Autodesk Inventor part; units mm, degrees
ref_plane "YZ Plane" through (0, 0, 0) normal (1, 0, 0) x (0, 1, 0)
ref_plane "XZ Plane" through (0, 0, 0) normal (0, 1, 0) x (-1, 0, 0)
ref_plane "XY Plane" through (0, 0, 0) normal (0, 0, 1) x (1, 0, 0)
sketch "Sketch1" plane through (0, 0, 0) normal (0, 0, 1) x (1, 0, 0)
  line L0 (0, 0) -> (71.1, 0)
  line L1 (71.1, 0) -> (71.1, 71.1)
  line L2 (71.1, 71.1) -> (0, 71.1)
  line L3 (0, 71.1) -> (0, 0)
  circle A0 centre (35.55, 35.55) radius 24.15
  dimension "d0" = 71.1
  dimension "d1" = 71.1
  dimension "d2" = 48.3
extrude "Extrusion1" add sketch "Sketch1" along normal blind 12.7
sketch "Sketch2" plane through (0, 0, 12.7) normal (0, 0, 1) x (1, 0, 0)
  line L0 (71.1, 71.1) -> (0, 71.1)
  line L1 (0, 71.1) -> (0, 0)
  line L2 (0, 0) -> (71.1, 0)
  line L3 (71.1, 0) -> (71.1, 71.1)
  circle A0 centre (35.55, 35.55) radius 24.15
  circle A1 centre (35.55, 35.55) radius 24.15
  circle A2 centre (35.55, 35.55) radius 32.4
  dimension "d5" = 64.8
extrude "Extrusion2" add sketch "Sketch2" along normal blind 7.9 contours A2
sketch "Sketch3" plane through (0, 71.1, 0) normal (0, 1, 0) x (1, 0, 0)
  line L0 (71.1, 0) -> (0, 0)
  line L1 (0, 0) -> (0, -12.7)
  line L2 (71.1, -12.7) -> (0, -12.7)
  line L3 (71.1, 0) -> (71.1, -12.7)
  line L4 (71.1, 0) -> (71.1, -12.7)
  line L5 (71.1, -12.7) -> (35.55, -12.7)
  line L6 (0, -12.7) -> (71.1, -12.7)
  line L7 (35.55, -12.7) -> (20.55, -12.7)
  line L8 (20.55, -12.7) -> (23.7, -12.7)
  arc A0 (23.7, -9.55) -> (20.55, -12.7) centre (23.7, -12.7) ccw
  line L9 (35.55, -12.7) -> (47.4, -12.7)
  arc A1 (50.55, -12.7) -> (47.4, -9.55) centre (47.4, -12.7) ccw
  line L10 (47.4, -9.55) -> (23.7, -9.55)
  dimension "d8" = 35.55
  dimension "d9" = 15
  dimension "d10" = 3.15
  dimension "d11" = 11.85
  dimension "d12" = 6.3
revolve "Revolution1" cut sketch "Sketch3" angle 360 about axis through (71.1, 71.1, 12.7) along (-1, 0, 0) contours L2 A0 L10 A1
sketch "Sketch4" plane through (0, 0, 12.7) normal (0, 0, 1) x (1, 0, 0)
  arc A0 (20.55, 71.1) -> (23.7, 67.95) centre (23.7, 71.1) ccw
  line L0 (20.55, 71.1) -> (0, 71.1)
  line L1 (0, 71.1) -> (0, 0)
  line L2 (0, 0) -> (71.1, 0)
  line L3 (71.1, 0) -> (71.1, 71.1)
  line L4 (71.1, 71.1) -> (50.55, 71.1)
  arc A1 (47.4, 67.95) -> (50.55, 71.1) centre (47.4, 71.1) ccw
  line L5 (47.4, 67.95) -> (35.55, 67.95)
  circle A2 centre (35.55, 35.55) radius 32.4
  line L6 (35.55, 67.95) -> (23.7, 67.95)
  line L7 (35.55, 35.55) -> (65.55, 35.55)
  line L8 (65.55, 35.55) -> (65.55, 65.55)
  line L9 (65.55, 65.55) -> (5.55, 65.55)
  line L10 (5.55, 65.55) -> (5.55, 5.55)
  line L11 (5.55, 5.55) -> (65.55, 5.55)
  circle A3 centre (65.55, 65.55) radius 3
  circle A4 centre (5.55, 65.55) radius 3
  circle A5 centre (5.55, 5.55) radius 3
  circle A6 centre (65.55, 5.55) radius 3
  dimension "d14" = 30
  dimension "d15" = 30
  dimension "d16" = 60
  dimension "d17" = 60
  dimension "d18" = 60
  dimension "d19" = 6
  dimension "d20" = 6
  dimension "d21" = 6
  dimension "d22" = 6
extrude "Extrusion3" cut sketch "Sketch4" against normal blind 12.7 contours A6 | A3 L8 L9 | L9 L8 A3 | A4 L10 L9 | L9 L10 A4 | A5 L11 L10 | L10 L11 A5
sketch "Sketch5" plane through (71.1, 0, 0) normal (1, 0, 0) x (0, 0, -1)
  line L0 (0, 0) -> (0, 71.1)
  line L1 (0, 71.1) -> (-12.7, 71.1)
  line L2 (-12.7, 0) -> (-12.7, 71.1)
  line L3 (0, 0) -> (-12.7, 0)
  line L4 (-12.7, 71.1) -> (-12.7, 0)
  line L5 (-12.7, 35.55) -> (-6.35, 35.55)
  circle A0 centre (-6.35, 35.55) radius 1
  line L6 (-6.35, 35.55) -> (-9.525, 35.55)
  line L7 (-9.525, 35.55) -> (-9.525, 65.55)
  line L8 (-9.525, 65.55) -> (-9.525, 61.97)
  line L9 (-9.525, 65.55) -> (-3.175, 65.55)
  line L10 (-3.175, 65.55) -> (-3.175, 5.55)
  line L11 (-3.175, 5.55) -> (-3.175, 9.13)
  line L12 (-3.175, 9.13) -> (-9.525, 9.13)
  circle A1 centre (-9.525, 9.13) radius 0.65
  circle A2 centre (-3.175, 9.13) radius 0.65
  circle A3 centre (-9.525, 61.97) radius 0.65
  circle A4 centre (-3.175, 61.97) radius 0.65
  line L13 (-9.525, 61.97) -> (-3.175, 61.97)
  dimension "d25" = 6.35
  dimension "d26" = 2
  dimension "d37" = 3.175
  dimension "d38" = 30
  dimension "d39" = 3.58
  dimension "d40" = 6.35
  dimension "d41" = 60
  dimension "d42" = 3.58
  dimension "d43" = 6.35
  dimension "d44" = 1.3
  dimension "d45" = 1.3
  dimension "d46" = 1.3
  dimension "d47" = 1.3
  dimension "d48" = 6.35
extrude "Extrusion4" cut sketch "Sketch5" against normal blind 4.75 contours A1 | A2 L10 | L10 L12 A2 | A3 L7 | L7 L13 A3 | A0 | L7 A3 L13 | L13 L10 A4 | A4 L10 L13 | A4 L10 | L10 A2 L12
sketch "Sketch6" plane through (0, 0, 0) normal (0, -1, 0) x (1, 0, 0)
  line L0 (0, 0) -> (71.1, 0)
  line L1 (71.1, 0) -> (71.1, 12.7)
  line L2 (0, 12.7) -> (71.1, 12.7)
  line L3 (0, 0) -> (0, 12.7)
  circle A0 centre (35.55, 6.35) radius 2
  dimension "d29" = 4
extrude "Extrusion5" cut sketch "Sketch6" against normal blind 6.1 contours A0
thread "Thread1"
chamfer "Chamfer1" distance 2.55 angle 45 4 edges at (71.1, 71.1, 6.35) (71.1, 0, 6.35) (0, 71.1, 6.35) (0, 0, 6.35)
sketch "Sketch7" plane through (0, 2.55, 0) normal (-1, 0, 0) x (0, 0, 1)
  circle A0 centre (9.525, 6.58) radius 0.65
  circle A1 centre (3.175, 6.58) radius 0.65
  circle A2 centre (3.175, 59.42) radius 0.65
  circle A3 centre (6.35, 33) radius 1
  circle A4 centre (9.525, 59.42) radius 0.65
  line L0 (0, 0) -> (12.7, 0)
  line L1 (0, 0) -> (0, 66)
  line L2 (12.7, 66) -> (0, 66)
  line L3 (12.7, 0) -> (12.7, 66)
  circle A5 centre (3.175, 59.42) radius 0.65
  circle A6 centre (9.525, 59.42) radius 0.65
  circle A7 centre (6.35, 33) radius 1
  circle A8 centre (3.175, 6.58) radius 0.65
  circle A9 centre (3.175, 6.58) radius 0.65
  circle A10 centre (9.525, 6.58) radius 0.65
  point P0 (0, -2.55)
  dimension "d49" = 1.3
  dimension "d50" = 1.3
  dimension "d51" = 2
  dimension "d52" = 1.3
  dimension "d53" = 1.3
extrude "Extrusion6" cut sketch "Sketch7" against normal blind 4.75 contours A0 | A1 | A2 | A3 | A4
properties part number "0x001" material "Iron, Cast"
Work out the finished part from the listing and answer in its coordinate system (mm). A direction names the side the tool comes from. Coordinates: 2 decimals unless noted, no trailing zeros. Write each loop counter-clockwise with the first axis right and the second up, starting at its lowest first coordinate (ties: lowest second). Pieces come first, ordered by that corner, then holes.
Q1. A cutting plane is placed at D-D, the plane y = 65.55. Give the vertices of the cut face in (x, z), then the cut area to 3 significant figures.
Q2. Determine the mould class of faces 1 (the face through (66.454, 25.818, 16.595)), 2 (the face through (2.342, 34.574, 6.133)), 3 (the face through (4.9, 62.62, 6.44)), 4 (the face through (11, 36, 0)) for opening direction Y: released by +Y, released by -Y, zero draft, split by the parting line, or undercut.
Q3. A cutting plane is placed at C-C, the plane y = 39. Give the vertices of the cut face in (x, z).
Q4. Which of the six approach directions +Z, -Z, +X, -X, +Y, -Y give full straight-line access (tool end or side, diameter ignored) to faces 5 (the face through (35.384, 68.897, 10.448)), 6 (the face through (36, 6.1, 6)), 7 (the face through (25, 4, 12.7)), 8 (the face through (4.75, 36, 6))?
Q5. A cutting plane is placed at B-B, the plane x = 58.5. Give the vertices of the cut face in (y, z), then the cut area to 3 significant figures.
Q6. Find the intervals of material crossed by line 1 (X direction, y = 65.55, z = 9); line 2 (Z direction, x = 1, y = 9); line 3 (Z direction, x = 68.5, y = 63), in increasing order.
Q7. Each of these flat-tipped pins is pushed along its axis until it touches: pin 1 Ø8 at (x, z) = (21.5, 10) entering from -Y; pin 2 Ø0.6 at (y, z) = (35.5, 6) entering from -X; pin 3 Ø3 at (y, z) = (15.5, 18) entering from -X; pin 4 Ø0.8 at (y, z) = (61.97, 9.525) entering from +X. Where does it stop, or does it pass through?
Q8. A cutting plane is placed at A-A, the plane z = 6.35. Give the vertices of the cut face in (x, y).
Findings below:
1. outline: (0, 0) - (2.55, 0) - (2.55, 12.7) - (0, 12.7) - close; (8.55, 0) - (62.55, 0) - (62.55, 12.7) - (47.79, 12.7) - (47.79, 20.6) - (23.31, 20.6) - (23.31, 12.7) - (8.55, 12.7) - close; (68.55, 0) - (71.1, 0) - (71.1, 12.7) - (68.55, 12.7) - close
1. area: 944 mm2
2. face 1: split by the parting line
2. face 2: undercut
2. face 3: undercut
2. face 4: zero draft
3. outline: (0, 0) - (11.65, 0) - (11.65, 20.6) - (3.33, 20.6) - (3.33, 12.7) - (0, 12.7) - close; (59.45, 0) - (71.1, 0) - (71.1, 12.7) - (67.77, 12.7) - (67.77, 20.6) - (59.45, 20.6) - close
4. face 5: +Z, +Y
4. face 6: -Y
4. face 7: +Z
4. face 8: -X
5. outline: (0, 0) - (28.03, 0) - (28.03, 20.6) - (12.68, 20.6) - (12.68, 12.7) - (0, 12.7) - close; (43.07, 0) - (71.1, 0) - (71.1, 12.7) - (58.42, 12.7) - (58.42, 20.6) - (43.07, 20.6) - close
5. area: 955 mm2
6. line 1: x = 0 to 2.55, 8.55 to 62.55, 68.55 to 71.1
6. line 2: z = 0 to 2.54, 3.81 to 8.89, 10.16 to 12.7
6. line 3: z = 0 to 12.7
7. pin 1: stops at y = 0
7. pin 2: stops at x = 4.75
7. pin 3: stops at x = 8.99
7. pin 4: stops at x = 66.35
8. outline: (0, 2.55) - (2.55, 0) - (33.55, 0) - (33.55, 6.1) - (37.55, 6.1) - (37.55, 0) - (68.55, 0) - (71.1, 2.55) - (71.1, 34.55) - (66.35, 34.55) - (66.35, 36.55) - (71.1, 36.55) - (71.1, 68.55) - (68.55, 71.1) - (2.55, 71.1) - (0, 68.55) - (0, 36.55) - (4.75, 36.55) - (4.75, 34.55) - (0, 34.55) - close; hole circle Ø6 at (5.55, 5.55); hole circle Ø6 at (5.55, 65.55); hole circle Ø48.3 at (35.55, 35.55); hole circle Ø6 at (65.55, 5.55); hole circle Ø6 at (65.55, 65.55)
